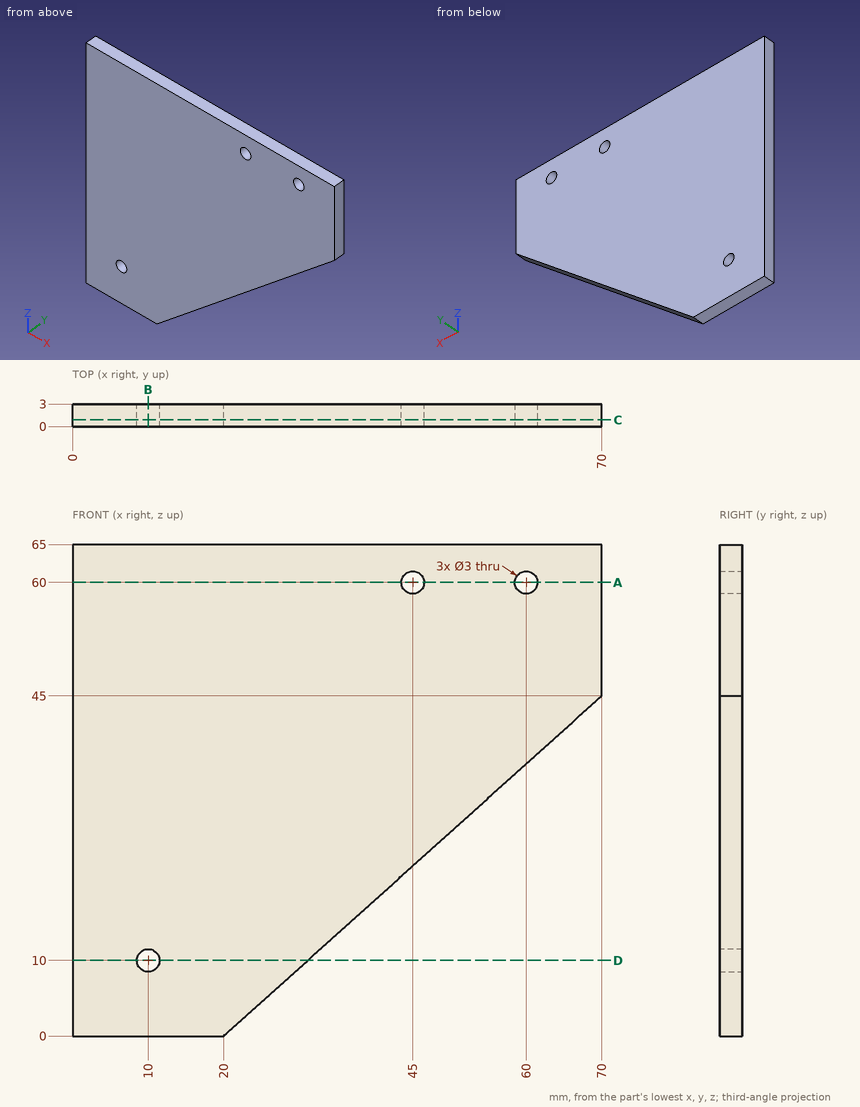
Study the drawing (mm; zero at the part's minimum x, y, z) and answer. Give positions to 0.01 mm unless a question says otherwise; leave off trailing zeros. Loops run counter-clockwise (first coordinate to the right, second up) from the corner with the lowest first, then second, coordinate; pieces in that order, holes last. Notation, with made-up numbers: (48.5, -24.5) -> (96.5, -24.5) arc R16 cw to (96.5, 0.5) -> close; hole circle Ø11 at (44, 50.5). An arc over 180 degrees is marked (long way). Use a Markdown table: item, result. Add a question column.
1) The part is cut by section D-D, the plane z = 10. Determine the outline of the cut face in (x, y), plus the area to 3 significant figures.
2) This flat-tipped pin is pushed along its axis until it touches: P1, Ø5, axis at x = 60, z = 60, coming from the -Y side. Where does it stop, or does it pass through?
3) The part is cut by section C-C, the plane y = 0.9. Determine the outline of the cut face in (x, z).
4) The part is cut by section B-B, the plane x = 10. Determine the outline of the cut face in (y, z), plus the area to 3 significant figures.
5) The part is cut by section A-A, the plane z = 60. Determine the outline of the cut face in (x, y), plus the area to 3 significant figures.
6) Consider line 1 along X through (y, z) = (2.3, 60); line 2 along X through (y, z) = (1.6, 10); line 3 along Z through (x, y) = (44.5, 0.5). Determine where each line is inside the solid, lowest interval first.
Reported:
| question | item | result |
|---|---|---|
| 1 | outline | (0, 0) -> (8.5, 0) -> (8.5, 3) -> (0, 3) -> close; (11.5, 0) -> (31.11, 0) -> (31.11, 3) -> (11.5, 3) -> close |
| 1 | area | 84.3 mm^2 |
| 2 | P1 | stops at y = 0 |
| 3 | outline | (0, 0) -> (20, 0) -> (70, 45) -> (70, 65) -> (0, 65) -> close; hole circle Ø3 at (10, 10); hole circle Ø3 at (45, 60); hole circle Ø3 at (60, 60) |
| 4 | outline | (0, 0) -> (3, 0) -> (3, 8.5) -> (0, 8.5) -> close; (0, 11.5) -> (3, 11.5) -> (3, 65) -> (0, 65) -> close |
| 4 | area | 186 mm^2 |
| 5 | outline | (0, 0) -> (43.5, 0) -> (43.5, 3) -> (0, 3) -> close; (46.5, 0) -> (58.5, 0) -> (58.5, 3) -> (46.5, 3) -> close; (61.5, 0) -> (70, 0) -> (70, 3) -> (61.5, 3) -> close |
| 5 | area | 192 mm^2 |
| 6 | line 1 | x = 0 to 43.5, 46.5 to 58.5, 61.5 to 70 |
| 6 | line 2 | x = 0 to 8.5, 11.5 to 31.11 |
| 6 | line 3 | z = 22.05 to 58.59, 61.41 to 65 |
